Input: part model. Units: mm. Frame: model coordinates. Coordinates: 2 decimals unless noted, no trailing zeros. Write each loop counter-clockwise with the first axis right and the second up, starting at its lowest first coordinate (ties: lowest second). Pieces come first, ordered by that corner, then holes.
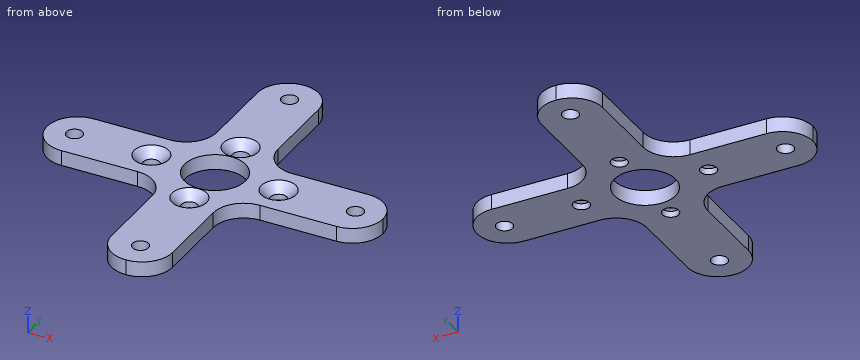
from build123d import *

# Parameters (mm, degrees)
SKETCH_1_R      = 1.6
SKETCH_1_R_2    = 6
EXTRUDE_1_DEPTH = 3
FILLET_1_R      = 6
CHAMFER_1_SIZE  = 1.8


with BuildPart() as part:
    # 草图1 → 凸台-拉伸1 (new body)
    with BuildSketch(Plane.XY):
        Polygon((-6, 0), (6, 0), (6, -27), (33, -27), (33, -39), (6, -39), (6, -66), (-6, -66), (-6, -39), (-33, -39), (-33, -27), (-6, -27), align=None)
        with Locations((0, -5.4)):
            Circle(SKETCH_1_R, mode=Mode.SUBTRACT)
        with Locations((-27.6, -33)):
            Circle(SKETCH_1_R, mode=Mode.SUBTRACT)
        with Locations((27.6, -33)):
            Circle(SKETCH_1_R, mode=Mode.SUBTRACT)
        with Locations((0, -60.6)):
            Circle(SKETCH_1_R, mode=Mode.SUBTRACT)
        with Locations((0, -23.5)):
            Circle(SKETCH_1_R, mode=Mode.SUBTRACT)
        with Locations((12.5, -33)):
            Circle(SKETCH_1_R, mode=Mode.SUBTRACT)
        with Locations((0, -42.5)):
            Circle(SKETCH_1_R, mode=Mode.SUBTRACT)
        with Locations((-12.5, -33)):
            Circle(SKETCH_1_R, mode=Mode.SUBTRACT)
        with Locations((0, -33)):
            Circle(SKETCH_1_R_2, mode=Mode.SUBTRACT)
    extrude(amount=EXTRUDE_1_DEPTH)

    # 圆角1
    fillet_1_edges = [part.edges().sort_by_distance(p)[0] for p in [
        (-6, -39, 1.5),
        (-6, -66, 1.5),
        (6, -66, 1.5),
        (6, -39, 1.5),
        (33, -39, 1.5),
        (33, -27, 1.5),
        (-6, 0, 1.5),
        (6, 0, 1.5),
        (6, -27, 1.5),
        (-6, -27, 1.5),
        (-33, -39, 1.5),
        (-33, -27, 1.5),
    ]]
    fillet(fillet_1_edges, radius=FILLET_1_R - 0.0001)  # a hair under: the kernel refuses the full size

    # 倒角1
    chamfer_1_edges = [part.edges().sort_by_distance(p)[0] for p in [
        (-1.6, -23.5, 3),
        (10.9, -33, 3),
        (-1.6, -42.5, 3),
        (-14.1, -33, 3),
    ]]
    chamfer(chamfer_1_edges, length=CHAMFER_1_SIZE)


solid = part.part
Item 1: Section query D-D, the plane y = -56.5. Return loops of the section in (x, z), then the cut area to 3 significant figures.
Item 2: Material intervals for line 1 (Y direction, x = 0, z = 0.8); line 2 (Y direction, x = 0, z = 2.15); line 3 (X direction, y = -8.5, z = 2.85), sorted ascending.
Item 3: Section query C-C, the plane x = -28. Return loops of the section in (y, z).
Item 4: Pin query (flat end, axial travel): pin 1 Ø5 at (x, y) = (-12.5, -33) entering from +Z; pin 2 Ø7 at (x, y) = (0, -33) entering from +Z; pin 3 Ø1.5 at (y, z) = (-50, 1.5) entering from +X; pin 4 Ø3.5 at (x, y) = (0, -23.5) entering from +Z. Return the tip coordinate at first contact, or that it passes through.
Item 5: Section query A-A, the plane z = 0.55. State how many separate pieces and enclosed holes the cut face has, then the cut area to 3 significant figures.
Item 6: Section query B-B, the plane y = -23.5. Return loops of the section in (x, z).
The answers:
1. outline: (-6, 0) - (6, 0) - (6, 3) - (-6, 3) - close
1. area: 36.0 mm2
2. line 1: y = -66 to -62.2, -59 to -44.1, -40.9 to -39, -27 to -25.1, -21.9 to -7, -3.8 to 0
2. line 2: y = -66 to -62.2, -59 to -45.05, -39.95 to -39, -27 to -26.05, -20.95 to -7, -3.8 to 0
2. line 3: x = -6 to 6
3. outline: (-38.92, 0) - (-34.55, 0) - (-34.55, 3) - (-38.92, 3) - close; (-31.45, 0) - (-27.08, 0) - (-27.08, 3) - (-31.45, 3) - close
4. pin 1: stops at z = 2.1
4. pin 2: passes through
4. pin 3: stops at x = 6
4. pin 4: stops at z = 1.35
5. separate pieces: 1
5. enclosed holes: 9
5. area: 1,230 mm2
6. outline: (-6.55, 0) - (-1.6, 0) - (-1.6, 1.2) - (-3.4, 3) - (-6.55, 3) - close; (1.6, 0) - (6.55, 0) - (6.55, 3) - (3.4, 3) - (1.6, 1.2) - close
